Design review of the part built by this model. Coordinates are the model's own, in mm. A direction names the side the tool comes from. Coordinates: 2 decimals unless noted, no trailing zeros. Write each loop counter-clockwise with the first axis right and the second up, starting at its lowest first coordinate (ties: lowest second). Pieces come first, ordered by that corner, then holes. Notation, with made-up numbers: (84.5, -20) - (89.5, -20) arc R17 ccw to (89.5, 13) - close; hole circle Ø2 at (68, 50.25). An arc over 180 degrees is marked (long way). Answer as CSV lines item,"result". Start each with the question number.
Q1. For line 1 along X through (y, z) = (412, -11); line 2 along X through (y, z) = (450.5, -9.75); line 3 along X through (y, z) = (38, -6.5), list the stretches that pass through material, from the lowest coordinate up. Write a range as [from, to].
Q2. Clearance check with flat-ended pins moving along their axes: pin 1 (6 mm diameter, centred on x = 461.5, z = 6, fed in from +Y); pin 2 (7.5 mm diameter, centred on y = 202.5, z = -0.5, fed in from -X); pin 3 (4 mm diameter, centred on x = 419.5, z = -5, fed in from +Y). State where each tip first meets the part, or that it passes through.
Q3. We need section A-A (z = 6.75). Write out the cut boundary in (x, y).
Q4. We need section B-B (x = 216). Write out the cut boundary in (y, z), plus the area to 3 significant figures.
Q5. Machinability: for faces 1 (the face through (309.036, 226.155, -0.178)), 2 (the face through (355, 268, -12.7)), 3 (the face through (646.52, 476.18, -0.18)), which of the approach directions +Z, -Z, +X, -X, +Y, -Y give a long, thin tool a straight path to every point of the face, cutting with its end or side? Answer none if there is none.
Q6. We need section C-C (y = 45.5). Write out the cut boundary in (x, z).
Q7. Mouldability with a two-part tool opening along Y and no side actions: class faces 4 (the face through (561.366, 437.421, -0.178)), 5 (the face through (713.667, 270, 0)), 6 (the face through (375, 25.4, 0)) as pulls with the +Y half, pulls with the -Y half, needs draft (parallel to the pull), parting line crosses it, or undercut.
Autodesk Inventor part; units mm, degrees
ref_plane "planeForPowerCells" through (-48.9804, 58.3726, 12.7) normal (-0.6428, 0.766, 0) x (0.766, 0.6428, 0)
ref_plane "planeForShootingPowerCells" through (528.484, 476.6081, 12.7) normal (-0.6428, 0.766, 0) x (0.766, 0.6428, 0)
ref_plane "Work Plane3" through (612.9122, 514.2944, 12.7) normal (0.766, 0.6428, 0) x (0, 0, -1)
sketch "Sketch1" plane through (0, 0, 0) normal (0, 0, 1) x (1, 0, 0)
  line L0 (0, 0) -> (544.8108, 457.1505)
  line L1 (0, 0) -> (749.0326, 0)
  line L2 (713.6671, 532.5231) -> (713.6671, 0)
  line L3 (713.6671, 532.5231) -> (577.4644, 418.2355)
  line L4 (577.4644, 418.2355) -> (544.8108, 457.1505)
  line L5 (69.7859, 25.4) -> (688.2671, 25.4)
  line L6 (688.2671, 25.4) -> (688.2671, 478.0527)
  line L7 (688.2671, 478.0527) -> (574.3337, 382.4512)
  line L8 (574.3337, 382.4512) -> (541.6801, 421.3662)
  line L9 (541.6801, 421.3662) -> (69.7859, 25.4)
  line L10 (688.2671, 511.21) -> (688.2671, 628.3123) construction
  line L11 (69.7859, 25.4) -> (39.5154, 0)
  line L12 (577.4644, 418.2355) -> (593.7912, 398.778) construction
  line L13 (688.2671, 25.4) -> (688.2671, 0) construction
  line L14 (688.2671, 25.4) -> (713.6671, 25.4) construction
  line L15 (541.6801, 421.3662) -> (525.3533, 440.8237) construction
  dimension "d10" = 40
  dimension "d14" = 177.8
  dimension "d15" = 711.2
  dimension "d16" = 50.8
  dimension "d17" = 25.4
  dimension "d18" = 25.4
  dimension "d19" = 25.4
  dimension "d20" = 25.4
  dimension "d21" = 25.4
  dimension "d33" = 50
  dimension "d36" = 76.2
  dimension "d40" = 618.4812
  dimension "d41" = 648.7517
  dimension "d42" = 688.2671
  dimension "d43" = 713.6671
  dimension "d44" = 452.6526
  dimension "d45" = 478.0527
  dimension "d46" = 507.1231
  dimension "d47" = 532.5231
  dimension "d48" = 685.8
extrude "Extrusion1" add sketch "Sketch1" along normal mid plane 25.4
ref_plane "planeForPowerCells" through (-48.9804, 58.3726, 12.7) normal (-0.6428, 0.766, 0) x (0.766, 0.6428, 0)
ref_plane "planeForShootingPowerCells" through (528.484, 476.6081, 12.7) normal (-0.6428, 0.766, 0) x (0.766, 0.6428, 0)
ref_plane "Work Plane3" through (612.9122, 514.2944, 12.7) normal (0.766, 0.6428, 0) x (0, 0, -1)
properties part number "ballRampWithPocketForPowerCell"
Results list:
1,line 1,"x = [491, 530.52], [549.54, 609.55], [688.27, 713.67]"
1,line 2,"x = [536.89, 550.39], [615.92, 655.43], [688.27, 713.67]"
1,line 3,"x = [45.29, 84.8], [688.27, 713.67]"
2,pin 1,"stops at y = 389.76"
2,pin 2,"stops at x = 236.86"
2,pin 3,"stops at y = 353.68"
3,outline,"(0, 0) - (713.67, 0) - (713.67, 532.52) - (577.46, 418.24) - (544.81, 457.15) - close; hole (69.79, 25.4) - (688.27, 25.4) - (688.27, 478.05) - (574.33, 382.45) - (541.68, 421.37) - close"
4,outline,"(0, -12.7) - (25.4, -12.7) - (25.4, 12.7) - (0, 12.7) - close; (148.09, -12.7) - (181.25, -12.7) - (181.25, 12.7) - (148.09, 12.7) - close"
4,area,"1,490 mm2"
5,face 1,"+Z, -Z"
5,face 2,"-Z, +X, -X, +Y, -Y"
5,face 3,"+Z, -Z, +Y"
6,outline,"(54.22, -12.7) - (93.74, -12.7) - (93.74, 12.7) - (54.22, 12.7) - close; (688.27, -12.7) - (713.67, -12.7) - (713.67, 12.7) - (688.27, 12.7) - close"
7,face 4,"pulls with the +Y half"
7,face 5,"needs draft"
7,face 6,"undercut"
